Autodesk Inventor part; units mm, degrees
ref_plane "YZ Plane" through (0, 0, 0) normal (1, 0, 0) x (0, 1, 0)
ref_plane "XZ Plane" through (0, 0, 0) normal (0, 1, 0) x (-1, 0, 0)
ref_plane "XY Plane" through (0, 0, 0) normal (0, 0, 1) x (1, 0, 0)
sketch "Skizze2" plane through (0, 0, 0) normal (0, 1, 0) x (-1, 0, 0)
  line L0 (14, 0) -> (-14, 0)
  line L1 (-14, 0) -> (-14, -5)
  line L2 (-14, -5) -> (1, -5)
  line L3 (1, -5) -> (1, -9)
  line L4 (1, -9) -> (14, -9)
  line L5 (14, -9) -> (14, 0)
  line L6 (0, -10.8) -> (0, 1.8)
  line L7 (19.6, 0) -> (-19.6, 0)
  point P0 (0, 0)
  dimension "d4" = 28
  dimension "d5" = 9
  dimension "d6" = 5
  dimension "d8" = 13
  dimension "d9" = 15
extrude "Extrusion2" add sketch "Skizze2" along normal blind 40
sketch "Skizze4" plane through (0, 40, 0) normal (0, 1, 0) x (1, 0, 0)
  line L0 (14, 5) -> (-1, 5)
  line L1 (-1, 5) -> (-1, 9)
  line L2 (-1, 9) -> (14, 9)
  line L3 (14, 9) -> (14, 5)
  line L4 (14, 5) -> (-1, 9) construction
  line L5 (-1, 5) -> (14, 9) construction
  line L6 (14, 5) -> (-1, 5)
  line L7 (-1, 5) -> (-1, 9)
  point P0 (0, 0)
  point P1 (6.5, 7)
extrude "Extrusion3" add sketch "Skizze4" against normal blind 22.5
sketch "Skizze6" plane through (14, 40, -9) normal (0, 0, -1) x (-1, 0, 0)
  line L0 (14, -48) -> (14, 8)
  line L1 (0, 0) -> (28, 0)
  point P0 (14, -40)
  point P1 (9.7574, -9.5074)
  point P2 (18.2426, -9.5074)
  point P3 (18.2426, -17.9926)
  point P4 (9.7574, -17.9926)
  dimension "d44" = 8.4853
  dimension "d45" = 8.4853
  dimension "d46" = 9.5074
  dimension "d47" = 17.9926
hole "Bohrung3" at (4.2426, 22.0074, -9) at (-4.2426, 30.4926, -9) direction (0, 0, 1) diameter 3 end through all
hole "Bohrung4" at (4.2426, 30.4926, -9) at (-4.2426, 22.0074, -9) direction (0, 0, 1) diameter 3.4 end through all counterbore diameter 6.5 counterbore depth 3.4
sketch "Skizze8" plane through (-14, 0, 0) normal (0, 0, 1) x (1, 0, 0)
  line L0 (0, 0) -> (0, 40)
  line L1 (28, 0) -> (28, 17.5)
  line L2 (0, 0) -> (28, 0)
  line L3 (28, 0) -> (28, 10)
  line L4 (28, 10) -> (0, 10)
  line L5 (0, 10) -> (0, 0)
  point P0 (14, 0)
  point P1 (0, 10)
  dimension "d85" = 10
extrude "Extrusion4" add sketch "Skizze8" along normal blind 25
sketch "Skizze9" plane through (14, 0, -5) normal (0, 0, -1) x (-1, 0, 0)
  line L0 (0, 0) -> (15, 0)
  line L1 (15, 0) -> (15, 17.5)
  line L2 (0, 0) -> (15, 0)
  line L3 (15, 0) -> (15, 17.5)
  line L4 (15, 17.5) -> (0, 17.5)
  line L5 (0, 17.5) -> (0, 0)
  point P0 (14, 0)
extrude "Extrusion5" add sketch "Skizze9" along normal blind 30
sketch "Skizze13" plane through (14, 0, -35) normal (0, 0, -1) x (-1, 0, 0)
  line L0 (0, 3.5) -> (0, 17.5)
  line L1 (15, 17.5) -> (0, 17.5)
  point P0 (14, 0)
  point P1 (11.95, 14.5)
  point P2 (11.95, 8.75)
  point P3 (6, 17.5)
  dimension "d102" = 11.95
  dimension "d103" = 3
  dimension "d104" = 8.75
hole "Bohrung7" at (2.05, 14.5, -35) at (2.05, 8.75, -35) direction (0, 0, 1) diameter 4 depth 6 tip angle 118
sketch "Skizze14" plane through (-1, 0, -9) normal (-1, 0, 0) x (0, 0, 1)
  line L0 (0, 0) -> (-26, 0)
  line L1 (-26, 0) -> (-26, 17.5)
  point P0 (9, 0)
  point P1 (-20, 3)
  point P2 (-5.5, 3)
  dimension "d112" = 3
  dimension "d113" = 6
  dimension "d114" = 14.5
hole "Bohrung8" at (-1, 3, -29) at (-1, 3, -14.5) direction (1, 0, 0) diameter 3.242 depth 8 tip angle 118
fillet "Rundung2" radius 1 1 edges at (-1, 8.75, -9)
sketch "Skizze15" plane through (-1, 17.5, -35) normal (0, 1, 0) x (1, 0, 0)
  circle A0 centre (12.5, 0) radius 3.45
  line L0 (15, -26) -> (15, 0)
  line L1 (0, 0) -> (15, 0)
  point P0 (1, -35)
  dimension "d123" = 6.9
  dimension "d124" = 2.5
extrude "Extrusion9" cut sketch "Skizze15" against normal through all
sketch "Skizze16" plane through (-2, 17.5, -9) normal (0, 1, 0) x (1, 0, 0)
  circle A0 centre (13.5, 26) radius 6
  arc A1 (10.05, 26) -> (16, 23.6225) centre (13.5, 26) ccw
  point P0 (2, -9)
  dimension "d127" = 12
extrude "Extrusion10" cut sketch "Skizze16" against normal blind 14
chamfer "Fasen3" distance 2 angle 45 1 edges at (10.2199, 3.5, -31.7963)
sketch "Skizze18" plane through (0, 0, 0) normal (0, -1, 0) x (1, 0, 0)
  circle A0 centre (11.5, -35) radius 3.95
  arc A1 (14, -32.6225) -> (8.05, -35) centre (11.5, -35) ccw
  point P0 (0, 0)
  dimension "d134" = 7.9
extrude "Extrusion11" cut sketch "Skizze18" against normal blind 1.25
properties part number "JH_int_Adapterplatte"
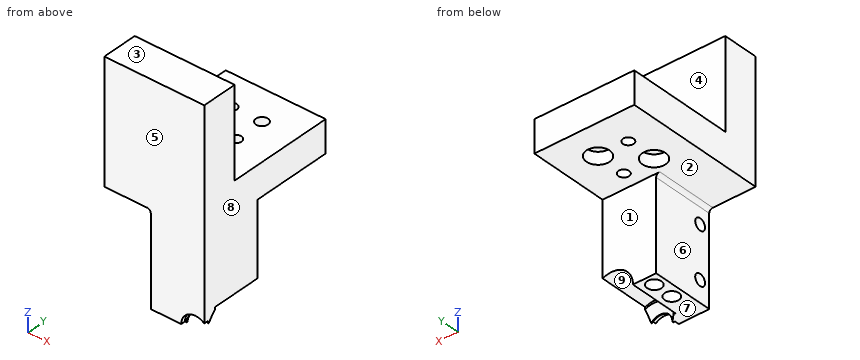
Check sheet for the modelled part. Datum: model origin and axes. Units: mm. Face numbers are marked on the shaded views. A direction names the side the tool comes from. Give positions to 0.01 mm unless a question says otherwise; leave off trailing zeros. Write each loop counter-clockwise with the first axis right and the second up, starting at its lowest first coordinate (ties: lowest second). Pieces come first, ordered by that corner, then holes. Notation, with made-up numbers: (41, 76.5) -> (64, 76.5) arc R23 cw to (64, 89.5) -> close; hole circle Ø4 at (9.25, 73.5). An arc over 180 degrees is marked (long way). Use CSV: the item, a comma, the result in double quotes. Start each with the question number.
Q1. Depth check by flat-ended pin: P1, Ø3, axis at x = 4.24, y = 30.49, coming from the -Z side; P2, Ø3.5, axis at x = 2.05, y = 8.75, coming from the -Z side; P3, Ø5, axis at x = -4.24, y = 22.01, coming from the -Z side; P4, Ø5, axis at y = 15.5, z = -26, coming from the -X side. Enter the tip coordinate at first touch or a pass-through.
Q2. Cross-section at B-B on y = 33. Enter the section's corners in (x, z), and give its area (3 significant figures).
Q3. Scan lines: line 1 along Y through (x, z) = (2.05, -33.7); line 2 along Z through (x, y) = (4.25, 3); line 3 along Y through (x, z) = (-3, -3.5). Record each from-to range of solid material in increasing order.
Q4. Cross-section at C-C on z = -8. Enter the section's corners in (x, y).
Q5. Tool access check on the marked faces 1, 2, 3, 4 and 5. Record the directions out of +Z, -Z, +X, -X, +Y, -Y that give a thin tool (end or side, any length) a straight path to the whole face; none if there is none.
Q6. Cross-section at A-A on z = 8. Enter the section's corners in (x, y).
Q7. Release check for a two-part mould opening along X. For the marked faces 6, 7, 8 and 9 record: +X half, -X half, draft (parallel to the pull), parting line (faces both ways), or undercut.
Working result:
1,P1,"passes through"
1,P2,"stops at z = -28.85"
1,P3,"stops at z = -5.6"
1,P4,"stops at x = -1"
2,outline,"(-14, -9) -> (2.17, -9) -> (2.17, -5.6) -> (6.31, -5.6) -> (6.31, -9) -> (14, -9) -> (14, 0) -> (-14, 0) -> close"
2,area,"238 mm^2"
3,line 1,"y = 0 to 6.75, 10.75 to 12.5, 16.5 to 17.5"
3,line 2,"z = -35 to -30.62, -27.38 to -16.12, -12.88 to 25"
3,line 3,"y = 0 to 20.85, 23.17 to 29.65, 31.33 to 40"
4,outline,"(-14, 0) -> (14, 0) -> (14, 40) -> (-14, 40) -> close; hole circle Ø6.5 at (-4.24, 22.01); hole circle Ø3 at (-4.24, 30.49); hole circle Ø6.5 at (4.24, 30.49); hole circle Ø3 at (4.24, 22.01)"
5,face 1,"-Z, +X, -X, +Y"
5,face 2,"-Z, -X, +Y"
5,face 3,"+Z, +X, -X, +Y, -Y"
5,face 4,"+Z, +X, -X, +Y"
5,face 5,"+Z, -Z, +X, -X, -Y"
6,outline,"(-14, 0) -> (14, 0) -> (14, 10) -> (-14, 10) -> close"
7,face 6,"-X half"
7,face 7,"draft"
7,face 8,"+X half"
7,face 9,"undercut"
